Could you check a few things on this model? Use its own coordinates, in mm. Give positions to 0.01 mm unless a question says otherwise; leave off trailing zeros. Loops run counter-clockwise (first coordinate to the right, second up) from the corner with the lowest first, then second, coordinate; pieces in that order, holes last. Notation, with made-up numbers: (-30.5, -31) - (17.5, -31) arc R27 ccw to (17.5, -2) - close; hole circle Ø4 at (-27, 12). An arc over 180 degrees is marked (long way). Write each question's results on one line, items separated by ' | '. Start each with the question number.
(1) I need wall thicknesses on line 1 (Z direction, x = 1, y = 67); line 2 (Y direction, x = -3, z = -39.5). Which ranges of each line are inside material? Lowest first, please.
(2) Suppose I cut it at D-D (z = -67.5). Please give me the cut outline in (x, y).
(3) For pin 1 (5 mm diameter, centred on x = -17.51, y = 63.55, fed in from -Z), with a flat end and sliding along its axis, tell me the tip position at first contact or that it passes through.
(4) Suppose I cut it at B-B (y = 64). Please give me the cut outline in (x, z), and give its area (3 significant figures).
(5) Suppose I cut it at C-C (x = 6). Please give me the cut outline in (y, z), and give its area (3 significant figures).
(6) If we mould it in two halves opening along X, with no side actions, what happens to faces 1 (the face through (-4, 57, -32.044)), 2 (the face through (-11, 44.1, -33.5)), 3 (the face through (-4.261, 54.875, -52.546))? For each: released by +X, released by -X, zero draft, split by the parting line, or undercut.
(7) Suppose I cut it at A-A (y = 42). Please give me the cut outline in (x, z).
from build123d import *

# Parameters (mm, degrees)
SKETCH2_R           = 21.5
SKETCH2_R_2         = 1.5
BOSS_EXTRUDE1_DEPTH = 3
SKETCH4_R           = 1.5
BOSS_EXTRUDE3_DEPTH = 35.5


with BuildPart() as part:
    # Sketch2 → Boss-Extrude1 (new body)
    with BuildSketch(Plane(origin=(-3.810522997, 56.305896335, -32.044001089), x_dir=(-0.4673428599090645, -0.8840761569525651, 0), z_dir=(0, 0, 1))):
        with Locations(Location((0, 0, 0), (0, 0, 27.861953602))):
            Circle(SKETCH2_R)
        with Locations(Location((0, 15.5, 0), (0, 0, 27.861953602))):
            Circle(SKETCH2_R_2, mode=Mode.SUBTRACT)
        with Locations(Location((15.5, 0, 0), (0, 0, 27.861953602))):
            Circle(SKETCH2_R_2, mode=Mode.SUBTRACT)
        with Locations(Location((0, -15.5, 0), (0, 0, 27.861953602))):
            Circle(SKETCH2_R_2, mode=Mode.SUBTRACT)
        with Locations(Location((-15.5, 0, 0), (0, 0, 27.861953602))):
            Circle(SKETCH2_R_2, mode=Mode.SUBTRACT)
    extrude(amount=-BOSS_EXTRUDE1_DEPTH)

    # Sketch4 → Boss-Extrude3 (add)
    with BuildSketch(Plane(origin=(0, 0, -35.044001089), x_dir=(-1, 0, 0), z_dir=(0, 0, -1))):
        with Locations(Location((3.810522997, 56.305896335, 0), (0, 0, 270))):
            Circle(SKETCH4_R)
    extrude(amount=BOSS_EXTRUDE3_DEPTH)


solid = part.part
Output values:
1) line 1: -35.04 to -32.04 | line 2: 55.04 to 57.57
2) outline: circle Ø3 at (-3.81, 56.31)
3) pin 1: z = -35.04
4) outline: (-23.89, -35.04) - (-18.94, -35.04) - (-18.94, -32.04) - (-23.89, -32.04) - close; (-16.08, -35.04) - (16.27, -35.04) - (16.27, -32.04) - (-16.08, -32.04) - close | area: 112 mm2
5) outline: (37.17, -35.04) - (75.44, -35.04) - (75.44, -32.04) - (37.17, -32.04) - close | area: 115 mm2
6) face 1: zero draft | face 2: undercut | face 3: split by the parting line
7) outline: (-19.86, -35.04) - (-12.43, -35.04) - (-12.43, -32.04) - (-19.86, -32.04) - close; (-9.68, -35.04) - (12.24, -35.04) - (12.24, -32.04) - (-9.68, -32.04) - close
